Read the model definition and answer for the solid it produces. Units are mm, in the model's axes. A direction names the side the tool comes from. Coordinates: 2 decimals unless noted, no trailing zeros. Write each loop counter-clockwise with the first axis right and the second up, starting at its lowest first coordinate (ties: lowest second). Pieces come first, ordered by that corner, then holes. Notation, with made-up numbers: (-31, -26) -> (4, -26) arc R36 ccw to (4, 10) -> close; hole circle Ø3 at (61.25, 30). An arc over 180 degrees is marked (long way). One line per item, written item: value. Start each with the question number.
1. Find section B-B, the plane x = 28.5. Write down the section's boundary in (y, z).
2. Find section D-D, the plane z = 6. Write down the section's boundary in (x, y).
3. For a pull along Y with two mould halves and no side action, classify faces 1 (the flat face through (0, -34, 3)), 2 (the cylindrical face through (0.215, 31.636, 1.129)), 3 (the flat face through (0, 20, 46)) as pulls with the +Y half, pulls with the -Y half, needs draft (parallel to the pull), parting line crosses it, or undercut.
4. Find section C-C, the plane y = -15. Write down the section's boundary in (x, z), and give its area (3 significant figures).
5. For faces 4 (the flat face through (0, -20, 46)), 5 (the flat face through (0, 34, 4)), 6 (the flat face through (0, 0, 90)), determine the directions among +Z, -Z, +X, -X, +Y, -Y from which every point of the face is accessible in a straight line to the end or side of a thin tool.
6. Find section A-A, the plane y = 30. Write down the section's boundary in (x, z).
7. Consider line 1 along Y through (x, z) = (0, 0.5); line 2 along Z through (x, y) = (0, 4.5); line 3 along X through (y, z) = (30, 1.8). Determine where each line is inside the solid, lowest interval first.
8. Given P1, Ø3, axis at x = -20.5, y = -21, coming from the -Z side; P2, Ø10, axis at x = 12, y = -29.5, coming from the +Z side; P3, Ø6, axis at x = 0.5, z = 50.5, coming from the -Y side; P4, Ø12, axis at x = 3.5, z = 55, coming from the +Y side, each flat-ended and moving along its own axis, determine where each tip first touches the part or whether it passes through.
```python
from build123d import *

# Parameters (mm, degrees)
F0_W            = 70
F0_H            = 40
F1_DEPTH        = 90
F3_DEPTH        = 40.001
F4_W            = 70
F4_H            = 3
F5_DEPTH        = 20
F6_W            = 70
F6_H            = 4
F7_DEPTH        = 20
F9_D            = 3.3
F9_DEPTH        = 12
F9_CSINK_D      = 6.72
F9_CSINK_ANGLE  = 90
F9_TIP          = 0.9914200214
F11_D           = 3.3
F11_DEPTH       = 12
F11_CSINK_D     = 6.72
F11_CSINK_ANGLE = 90
F11_TIP         = 0.9914200214


with BuildPart() as f1:
    # F0 (on Top) → F1 (new body)
    with BuildSketch(Plane.XY):
        Rectangle(F0_W, F0_H)
    extrude(amount=F1_DEPTH)

    # F2 (on face) → F3 (cut, through all)
    with BuildSketch(Plane(origin=(0, 20, 0), x_dir=(-1, 0, 0), z_dir=(0, 1, 0))):
        with BuildLine():
            ThreePointArc((0, 68.5), (6.0104076401, 70.9895923599), (8.5, 77))
            ThreePointArc((8.5, 77), (-6.0104076401, 83.0104076401), (0, 68.5))
        make_face()
    extrude(amount=-F3_DEPTH, mode=Mode.SUBTRACT)

    # F4 (on face) → F5 (join)
    with BuildSketch(Plane.XZ.offset(20)):
        with Locations((0, 1.5)):
            Rectangle(F4_W, F4_H)
    extrude(amount=F5_DEPTH)

    # F6 (on face) → F7 (join)
    with BuildSketch(Plane(origin=(0, 20, 0), x_dir=(-1, 0, 0), z_dir=(0, 1, 0))):
        with Locations((0, 2)):
            Rectangle(F6_W, F6_H)
    extrude(amount=F7_DEPTH)

    # F9
    with Locations(Plane.XY.offset(3)):
        with Locations((0, -30)):
            CounterSinkHole(F9_D / 2, F9_CSINK_D / 2, depth=F9_DEPTH, counter_sink_angle=F9_CSINK_ANGLE)
            with Locations((0, 0, -(F9_DEPTH + F9_TIP / 2))):  # 118° drill point
                Cone(0, F9_D / 2, F9_TIP, mode=Mode.SUBTRACT)

    # F11
    with Locations(Plane.XY.offset(4)):
        with Locations((0, 30)):
            CounterSinkHole(F11_D / 2, F11_CSINK_D / 2, depth=F11_DEPTH, counter_sink_angle=F11_CSINK_ANGLE)
            with Locations((0, 0, -(F11_DEPTH + F11_TIP / 2))):  # 118° drill point
                Cone(0, F11_D / 2, F11_TIP, mode=Mode.SUBTRACT)


solid = f1.part
```
Answer block:
1. outline: (-40, 0) -> (40, 0) -> (40, 4) -> (20, 4) -> (20, 90) -> (-20, 90) -> (-20, 3) -> (-40, 3) -> close
2. outline: (-35, -20) -> (35, -20) -> (35, 20) -> (-35, 20) -> close
3. face 1: needs draft
3. face 2: undercut
3. face 3: pulls with the +Y half
4. outline: (-35, 0) -> (35, 0) -> (35, 90) -> (-35, 90) -> close; hole circle Ø17 at (0, 77)
4. area: 6,070 mm2
5. face 4: +Z, +X, -X, -Y
5. face 5: +Z, +X, -X, +Y
5. face 6: +Z, +X, -X, +Y, -Y
6. outline: (-35, 0) -> (-1.65, 0) -> (-1.65, 2.29) -> (-3.36, 4) -> (-35, 4) -> close; (1.65, 0) -> (35, 0) -> (35, 4) -> (3.36, 4) -> (1.65, 2.29) -> close
7. line 1: y = -40 to -31.65, -28.35 to 28.35, 31.65 to 40
7. line 2: z = 0 to 68.5, 85.5 to 90
7. line 3: x = -35 to -1.65, 1.65 to 35
8. P1: stops at z = 0
8. P2: stops at z = 3
8. P3: stops at y = -20
8. P4: stops at y = 20
